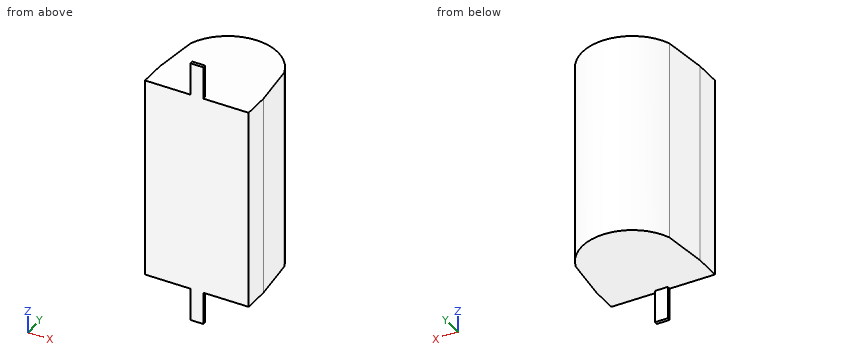
```python
from build123d import *

# Parameters (mm, degrees)
F1_DEPTH = 31
F2_W     = 2
F2_H     = 0.5
F3_DEPTH = 5
F4_W     = 2
F4_H     = 0.5
F5_DEPTH = 5


with BuildPart() as f1:
    # F0 (on Top) → F1 (new body)
    with BuildSketch(Plane.XY):
        with BuildLine():
            Line((-8, 3.136335), (8, 3.136335))
            Line((8, 3.136335), (8, 7.136335))
            Line((8, 7.136335), (7.222222, 14.092991))
            ThreePointArc((7.222222, 14.092991), (0, 19.136335), (-7.222222, 14.092991))
            Line((-7.222222, 14.092991), (-8, 7.136335))
            Line((-8, 7.136335), (-8, 3.136335))
        make_face()
    extrude(amount=F1_DEPTH)

    # F2 (on face) → F3 (join)
    with BuildSketch(Plane.XY.offset(31)):
        with Locations((0, 3.386335)):
            Rectangle(F2_W, F2_H)
    extrude(amount=F3_DEPTH)

    # F4 (on face) → F5 (join)
    with BuildSketch(Plane(origin=(0, 0, 0), x_dir=(1, 0, 0), z_dir=(0, 0, -1))):
        with Locations((0, -3.386335)):
            Rectangle(F4_W, F4_H)
    extrude(amount=F5_DEPTH)


solid = f1.part
```
For this review, take the finished solid that the model builds, in its own axes (mm). Give positions to 0.01 mm unless a question says otherwise; leave off trailing zeros. Order: outer loops, then holes, each group sorted by start corner. A loop starts at its lowest first (then second) coordinate and runs counter-clockwise, first axis right, second up.
1) Wall thickness on line 1 (Z direction, x = -5.5, y = 14.75); line 2 (Y direction, x = -0.25, z = 31.5); line 3 (Y direction, x = 6, z = 20.5): over which ranges is each line inside the solid? List them lowest first.
2) Take a section at A-A (y = 5.5). Give the boundary of the cut face in (x, z).
3) Take a section at D-D (y = 12.25). Give the boundary of the cut face in (x, z), then the cut area to 3 significant figures.
4) Insertion check: pin 1 (0.6 mm diameter, centred on x = 0.5, z = -1.5, fed in from +Y); pin 2 (5 mm diameter, centred on x = 0, y = 13.5, fed in from -Z); pin 3 (5 mm diameter, centred on y = 12.5, z = 17.5, fed in from -X). Each pin has a flat end and moves straight along its axis. Give the tip position at first contact, or say it passes through.
5) Take a section at B-B (z = 27). Give the boundary of the cut face in (x, y).
6) Take a section at C-C (x = -0.5). Give the boundary of the cut face in (y, z), then the cut area to 3 significant figures.
Derived:
1. line 1: z = 0 to 31
1. line 2: y = 3.14 to 3.64
1. line 3: y = 3.14 to 16.26
2. outline: (-8, 0) - (8, 0) - (8, 31) - (-8, 31) - close
3. outline: (-7.43, 0) - (7.43, 0) - (7.43, 31) - (-7.43, 31) - close
3. area: 461 mm2
4. pin 1: stops at y = 3.64
4. pin 2: stops at z = 0
4. pin 3: stops at x = -7.68
5. outline: (-8, 3.14) - (8, 3.14) - (8, 7.14) - (7.22, 14.09) arc R7.69 ccw to (-7.22, 14.09) - (-8, 7.14) - close
6. outline: (3.14, -5) - (3.64, -5) - (3.64, 0) - (19.12, 0) - (19.12, 31) - (3.64, 31) - (3.64, 36) - (3.14, 36) - close
6. area: 500 mm2
